CAD build for the part. Positions are in the model's coordinates, mm. A direction names the side the tool comes from. Round coordinates to 2 decimals unless told otherwise and drop trailing zeros. Order: outer loops, then holes, each group sorted by start corner. A loop starts at its lowest first (then second) coordinate and runs counter-clockwise, first axis right, second up.
Autodesk Inventor part; units mm, degrees
ref_plane "YZ Plane" through (0, 0, 0) normal (1, 0, 0) x (0, 1, 0)
ref_plane "XZ Plane" through (0, 0, 0) normal (0, 1, 0) x (-1, 0, 0)
ref_plane "XY Plane" through (0, 0, 0) normal (0, 0, 1) x (1, 0, 0)
sketch "Esquisse1" plane through (0, 0, 0) normal (0, 0, 1) x (1, 0, 0)
  line L0 (-6, -5) -> (6, -5)
  line L1 (6, -5) -> (6, 5)
  line L2 (6, 5) -> (-6, 5)
  line L3 (-6, 5) -> (-6, -5)
  point P0 (0, 0)
  dimension "d0" = 10
  dimension "d1" = 12
  dimension "d2" = 6
  dimension "d3" = 5
extrude "Extrusion1" add sketch "Esquisse1" along normal blind 9
sketch "Esquisse2" plane through (0, 0, 9) normal (0, 0, 1) x (1, 0, 0)
  circle A0 centre (0, 0) radius 2
  dimension "d6" = 4
extrude "Extrusion2" add sketch "Esquisse2" along normal blind 1
fillet "Congé1" radius 1 4 edges at (-6, 5, 4.5) (6, 5, 4.5) (6, -5, 4.5) (-6, -5, 4.5)
properties part number "reducteur" material "Laiton, jaune doux"
1. Cut at D-D, the plane x = -3. Write the cut outline in (y, z), and give its area (3 significant figures).
2. Cut at A-A, the plane y = 0. Write the cut outline in (x, z), and give its area (3 significant figures).
3. Cut at C-C, the plane z = 9.5. Write the cut outline in (x, y).
4. Tool access for faces 1 (the face through (-0.434, 1.952, 9.493)), 2 (the face through (0, 0, 0)): list every direction of +Z, -Z, +X, -X, +Y, -Y with a clear straight run to the whole face (end or side of a thin tool).
5. Drill centre lines: line 1 (Z direction, x = -3.5, y = 1); line 2 (X direction, y = 4.25, z = 0.75). Where is each one in solid material? Low to high.
6. Pin check, flat tip, straight feed: P1, Ø1, axis at x = 4.5, y = -3.5, coming from the +Z side. Stop position of the tip, or through.
7. Cut at B-B, the plane x = 0. Write the cut outline in (y, z).
Outcome:
1. outline: (-5, 0) - (5, 0) - (5, 9) - (-5, 9) - close
1. area: 90.0 mm2
2. outline: (-6, 0) - (6, 0) - (6, 9) - (2, 9) - (2, 10) - (-2, 10) - (-2, 9) - (-6, 9) - close
2. area: 112 mm2
3. outline: circle Ø4 at (0, 0)
4. face 1: +Z
4. face 2: -Z, +X, -X, +Y, -Y
5. line 1: z = 0 to 9
5. line 2: x = -5.97 to 5.97
6. P1: stops at z = 9
7. outline: (-5, 0) - (5, 0) - (5, 9) - (2, 9) - (2, 10) - (-2, 10) - (-2, 9) - (-5, 9) - close
